from build123d import *

# Parameters (mm, degrees)
ESQUISSE1_R                  = 19.25
ESQUISSE1_R_2                = 2.5
BOSS_EXTRU_1_DEPTH           = 42
ENL_V_MAT_EXTRU_1_DEPTH      = 74.881298321
ENL_V_MAT_EXTRU_1_DEPTH_BACK = 74.881298321
ESQUISSE2_W                  = 90
ESQUISSE2_H                  = 30
ESQUISSE3_R                  = 1
ENL_V_MAT_EXTRU_2_DEPTH      = 42


with BuildPart() as part:
    # Esquisse1 → Boss.-Extru.1 (new body)
    with BuildSketch(Plane.XY):
        with BuildLine():
            Line((12.13875, 26.612276273), (53.5275, 7.733481994))
            ThreePointArc((53.5275, 7.733481994), (58.5, 0), (53.5275, -7.733481994))
            Line((53.5275, -7.733481994), (12.13875, -26.612276273))
            ThreePointArc((12.13875, -26.612276273), (-29.25, 0), (12.13875, 26.612276273))
        make_face()
        with Locations(Location((0, 0, 0), (0, 0, 180))):
            Circle(ESQUISSE1_R, mode=Mode.SUBTRACT)
        with Locations(Location((50, 0, 0), (0, 0, 180))):
            Circle(ESQUISSE1_R_2, mode=Mode.SUBTRACT)
    extrude(amount=BOSS_EXTRU_1_DEPTH)

    # Esquisse2 → Enlèv. mat.-Extru.1 (cut, two sides: drawn at the far end of the back side and taken through both)
    with BuildSketch(Plane(origin=(5.218823759, 0, 0), x_dir=(1, 0, 0), z_dir=(0, 1, 0)).offset(-ENL_V_MAT_EXTRU_1_DEPTH_BACK)):
        with Locations((-11.691323759, -21)):
            Rectangle(ESQUISSE2_W, ESQUISSE2_H)
    extrude(amount=ENL_V_MAT_EXTRU_1_DEPTH + ENL_V_MAT_EXTRU_1_DEPTH_BACK, mode=Mode.SUBTRACT)

    # Esquisse3 → Enlèv. mat.-Extru.2 (cut)
    with BuildSketch(Plane.XY.offset(42)):
        with Locations((45, 5)):
            Circle(ESQUISSE3_R)
        with Locations((45, -5)):
            Circle(ESQUISSE3_R)
        with Locations((-15, 19)):
            Circle(ESQUISSE3_R)
        with Locations((-15, -19)):
            Circle(ESQUISSE3_R)
    extrude(amount=-ENL_V_MAT_EXTRU_2_DEPTH, mode=Mode.SUBTRACT)


solid = part.part
Geometry: final body of the model. Coordinates: model frame, mm. A direction names the side the tool comes from. Round coordinates to 2 decimals unless told otherwise and drop trailing zeros. Write each loop counter-clockwise with the first axis right and the second up, starting at its lowest first coordinate (ties: lowest second). Pieces come first, ordered by that corner, then holes. Notation, with made-up numbers: M 29.5,4 L 49.5,4 A27 ccw 49.5,31 Z; hole C 27.25,88 d7. An arc over 180 degrees is marked long. Write item = value, one per line.
Item 1: Section query D-D on y = -13.5. Return loops of the section in (x, z).
Findings:
outline = M -25.95,0 L -13.72,0 L -13.72,6 L -25.95,6 Z; M -25.95,36 L -13.72,36 L -13.72,42 L -25.95,42 Z; M 13.72,0 L 40.89,0 L 40.89,42 L 13.72,42 L 13.72,36 L 38.53,36 L 38.53,6 L 13.72,6 Z
Item 2: Section query A-A on x = 0. Return loops of the section in (y, z), then the cut area to 3 significant figures.
Findings:
outline = M -29.25,0 L -19.25,0 L -19.25,6 L -29.25,6 Z; M -29.25,36 L -19.25,36 L -19.25,42 L -29.25,42 Z; M 19.25,0 L 29.25,0 L 29.25,6 L 19.25,6 Z; M 19.25,36 L 29.25,36 L 29.25,42 L 19.25,42 Z
area = 240 mm^2
Item 3: Pull-direction query (X, two-part tool) for faces 1 (the face through (-29.24, -0.82, 38.96)), 2 (the face through (-15, 18, 3)), 3 (the face through (15.28, 11.71, 38.96)), 4 (the face through (25, 0, 42)); classes: pulls with the +X half, pulls with the -X half, needs draft (parallel to the pull), parting line crosses it, or undercut.
Findings:
face_1 = parting line crosses it
face_2 = undercut
face_3 = undercut
face_4 = needs draft
Item 4: Section query C-C on z = 26. Return loops of the section in (x, y).
Findings:
outline = M 38.53,-14.58 L 53.53,-7.73 A8.5 ccw 53.53,7.73 L 38.53,14.58 Z; hole C 45,-5 d2; hole C 45,5 d2; hole C 50,0 d5
Item 5: Section query B-B on y = 0. Return loops of the section in (x, z), then the cut area to 3 significant figures.
Findings:
outline = M -29.25,0 L -19.25,0 L -19.25,6 L -29.25,6 Z; M -29.25,36 L -19.25,36 L -19.25,42 L -29.25,42 Z; M 19.25,0 L 47.5,0 L 47.5,42 L 19.25,42 L 19.25,36 L 38.53,36 L 38.53,6 L 19.25,6 Z; M 52.5,0 L 58.5,0 L 58.5,42 L 52.5,42 Z
area = 980 mm^2
Item 6: Material intervals for line 1 along Z through (x, y) = (18.5, -7); line 2 along Y through (x, z) = (0, 38.55); line 3 along Y through (x, z) = (-15, 40.7), sorted ascending. Write a range as [from, to].
Findings:
line_1 = [0, 6], [36, 42]
line_2 = [-29.25, -19.25], [19.25, 29.25]
line_3 = [-25.11, -20], [-18, -12.06], [12.06, 18], [20, 25.11]
Item 7: Pin query (flat end, axial travel): P1, Ø1.2, axis at x = -15, y = -19, coming from the -Z side; P2, Ø14.5, axis at y = 4, z = 16.5, coming from the -X side. Return the tip coordinate at first contact, or that it passes through.
Findings:
P1 = through
P2 = 38.53
Item 8: Access query for faces 5 (the face through (41.74, 13.11, 20.71)), 6 (the face through (38.528, 0, 21)). Directions: +Z, -Z, +X, -X, +Y, -Y. A direction counts if a zero-diameter tool reaches every point of the face in a straight line with its end or side. Return the directions, or none.
Findings:
face_5 = +Z, -Z, +X, +Y
face_6 = -X, +Y, -Y
